from build123d import *

# Parameters (mm, degrees)
SKETCH_1_W      = 60
SKETCH_1_H      = 60
EXTRUDE_1_DEPTH = 20


with BuildPart() as part:
    # 草图2 for 放样1 → 放样1 section 0
    with BuildSketch(Plane.XY.offset(50)):
        with BuildLine():
            # circular arc as an exact rational Bezier (weights 1, cos(half-angle), 1)
            Bezier((106.066017178, 106.066017178), (0, 212.132034356), (-106.066017178, 106.066017178), weights=[1, 0.707106781, 1])
            Bezier((-106.066017178, 106.066017178), (-212.132034356, 0), (-106.066017178, -106.066017178), weights=[1, 0.707106781, 1])
            Bezier((-106.066017178, -106.066017178), (0, -212.132034356), (106.066017178, -106.066017178), weights=[1, 0.707106781, 1])
            Bezier((106.066017178, -106.066017178), (212.132034356, 0), (106.066017178, 106.066017178), weights=[1, 0.707106781, 1])
        make_face()
    # 草图1 → 放样1 section 1
    with BuildSketch(Plane.XY):
        Rectangle(SKETCH_1_W, SKETCH_1_H)
    loft()

    # 草图3 → 凸台-拉伸1 (add)
    with BuildSketch(Plane.XY.offset(50)):
        with BuildLine():
            ThreePointArc((-106.066017178, -106.066017178), (0, -150), (106.066017178, -106.066017178))
            ThreePointArc((106.066017178, -106.066017178), (150, 0), (106.066017178, 106.066017178))
            ThreePointArc((106.066017178, 106.066017178), (0, 150), (-106.066017178, 106.066017178))
            ThreePointArc((-106.066017178, 106.066017178), (-150, 0), (-106.066017178, -106.066017178))
        make_face()
    extrude(amount=EXTRUDE_1_DEPTH)


solid = part.part
Check sheet for the modelled part. Datum: model origin and axes. Units: mm. Coordinates: 2 decimals unless noted, no trailing zeros. Loops run counter-clockwise (first coordinate to the right, second up) from the corner with the lowest first, then second, coordinate; pieces in that order, holes last. Notation, with made-up numbers: (80.25, 31) -> (123.25, 31) arc R22 cw to (123.25, 70) -> close; hole circle Ø4 at (67, 35.25). An arc over 180 degrees is marked (long way). Write item = value, one per line. Start each with the question number.
1. Section check A-A on z = 58. Record the cut outline in (x, y).
2. Draft check along X on faces 1 (the flat face through (-2, 2, 70)), 2 (the cylindrical face through (-133.027, 69.309, 59.86)). Enter one of: released by +X, released by -X, zero draft, split by the parting line, or undercut.
3. Material ranges on line 1 (Y direction, x = -23, z = 23); line 2 (Y direction, x = -138, z = 67); line 3 (X direction, y = -35.5, z = 11.5), recorded low to high.
4. Depth check by flat-ended pin: P1, Ø2, axis at x = -33, y = -79.5, coming from the -Z side; P2, Ø3, axis at x = 38.5, z = 53, coming from the +Y side; P3, Ø5, axis at y = 26.5, z = 60, coming from the +X side. Enter the tip coordinate at first touch or a pass-through.
Responses:
q1.outline = circle Ø300 at (0, 0)
q2.face_1 = zero draft
q2.face_2 = split by the parting line
q3.line_1 = -82.85 to 82.85
q3.line_2 = -58.79 to 58.79
q3.line_3 = -51.97 to 51.97
q4.P1 = 22.24
q4.P2 = 145.37
q4.P3 = 148.07
